Verification items for this drawing (mm, ordinates from the low corner). A direction names the side the tool comes from. Coordinates: 2 decimals unless noted, no trailing zeros. Write each loop counter-clockwise with the first axis right and the second up, starting at its lowest first coordinate (ties: lowest second). Pieces come first, ordered by that corner, then holes. Notation, with made-up numbers: M 27,6 L 58,6 A33 ccw 58,43 Z; hole C 69.5,88 d9. An arc over 180 degrees is marked long. Answer as CSV lines item,"result". Start each with the question number.
1) Section check C-C (x = 2.35). Record the cut outline in (y, z).
2) Material ranges on L1, parallel to Z at x = 2.5, y = 8.5; L2, parallel to Y at x = 0.45, z = 6; L3, parallel to Z at x = 3.6, y = 9.5, recorded low to high. Write a range as [from, to].
3) Section check D-D (y = 15.5). Record the cut outline in (x, z).
4) Section check A-A (z = 8.5). Record the cut outline in (x, y).
5) Access from +Z, -Z, +X, -X, +Y, -Y to the whole of each face (thin tool, end or side, straight path). Record for the marked faces 3 and 4.
6) Draft check along Z on the marked faces 1 and 2. Enter one of: +Z half, -Z half, draft (parallel to the pull), parting line (faces both ways), or undercut.
7) Go/stop test with flat-tipped pins: pin 1 Ø6 at (y, z) = (4.5, 12) entering from +X; pin 2 Ø1 at (x, z) = (3.5, 7.5) entering from -Y; pin 3 Ø2 at (x, z) = (3.5, 11) entering from -Y; pin 4 Ø1.5 at (x, y) = (2, 10) entering from -Z. Record where each tip stops, or that it passes through.
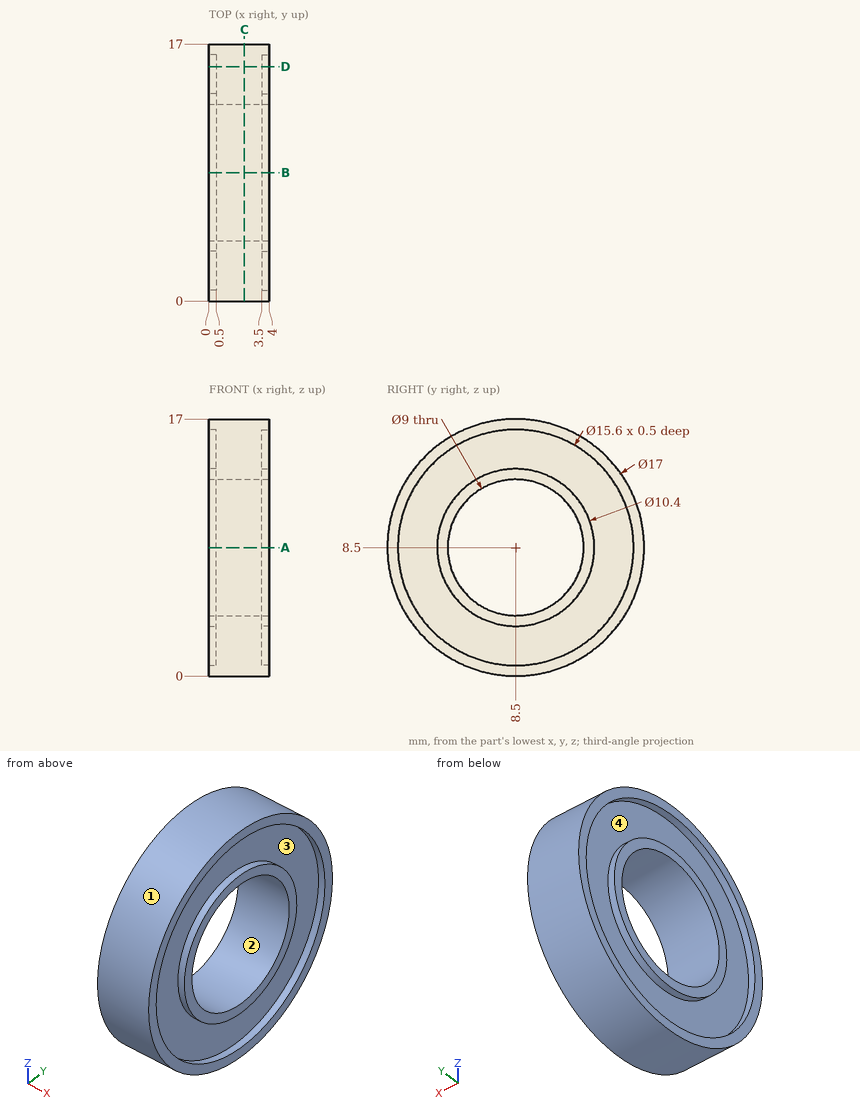
Results found:
1,outline,"C 8.5,8.5 d17; hole C 8.5,8.5 d9"
2,L1,"z = [0, 4], [13, 17]"
2,L2,"y = [0.38, 1.11], [3.94, 4.76], [12.24, 13.06], [15.89, 16.62]"
2,L3,"z = [0.06, 0.76], [3.4, 4.11], [12.89, 13.6], [16.24, 16.94]"
3,outline,"M 0,3.68 L 4,3.68 L 4,5.06 L 3.5,5.06 L 3.5,11.94 L 4,11.94 L 4,13.32 L 0,13.32 L 0,11.94 L 0.5,11.94 L 0.5,5.06 L 0,5.06 Z"
4,outline,"M 0,0 L 4,0 L 4,0.7 L 3.5,0.7 L 3.5,3.3 L 4,3.3 L 4,4 L 0,4 L 0,3.3 L 0.5,3.3 L 0.5,0.7 L 0,0.7 Z; M 0,13 L 4,13 L 4,13.7 L 3.5,13.7 L 3.5,16.3 L 4,16.3 L 4,17 L 0,17 L 0,16.3 L 0.5,16.3 L 0.5,13.7 L 0,13.7 Z"
5,face 3,"+X"
5,face 4,"-X"
6,face 1,"parting line"
6,face 2,"undercut"
7,pin 1,"stops at x = 4"
7,pin 2,"stops at y = 0.01"
7,pin 3,"stops at y = 0.13"
7,pin 4,"stops at z = 0.03"
